```python
from build123d import *

# Parameters (mm, degrees)
F0_R     = 25
F1_DEPTH = 20
F2_R     = 14
F3_DEPTH = 4
F2_R_2   = 25
F2_R_3   = 16.4
F4_DEPTH = 10
F5_SIZE  = 5


with BuildPart() as f1:
    # F0 (on Top) → F1 (new body)
    with BuildSketch(Plane.XY):
        Circle(F0_R)
    extrude(amount=F1_DEPTH)

    # F2 (on face) → F3 (join)
    with BuildSketch(Plane.XY.offset(20)):
        Circle(F2_R)
    extrude(amount=F3_DEPTH)

    # F2 (on face) → F4 (join)
    with BuildSketch(Plane.XY.offset(20)):
        Circle(F2_R_2)
        Circle(F2_R_3, mode=Mode.SUBTRACT)
    extrude(amount=F4_DEPTH)

    # F5
    f5_edges = [f1.edges().sort_by_distance(p)[0] for p in [
        (-25, 0, 0),
    ]]
    chamfer(f5_edges, length=F5_SIZE)


solid = f1.part
```
Input: part model. Units: mm. Frame: model coordinates. A direction names the side the tool comes from. Coordinates: 2 decimals unless noted, no trailing zeros. Write each loop counter-clockwise with the first axis right and the second up, starting at its lowest first coordinate (ties: lowest second). Pieces come first, ordered by that corner, then holes. Notation, with made-up numbers: M 29,28.5 L 52,28.5 A20 cw 52,40.5 Z; hole C 89,77.25 d4. An arc over 180 degrees is marked long. Use one line per item in the form item = value.
Q1. Material intervals for probe 1 along Y at (x, z) = (0, 22.25); probe 2 along Y at (x, z) = (0, 27); probe 3 along X at (y, z) = (-11, 20.25), sorted ascending. Write a range as from..to.
Answer below:
probe_1 = -25..-16.4, -14..14, 16.4..25
probe_2 = -25..-16.4, 16.4..25
probe_3 = -22.45..-12.16, -8.66..8.66, 12.16..22.45
Q2. Draft query along X for faces 3 (the face through (12.932, -5.362, 21.972)), 4 (the face through (0, 0, 24)), 5 (the face through (0, 0, 0)), 6 (the face through (-4.39, -19.76, 0.24)). Return one class per face: released by +X, released by -X, zero draft, split by the parting line, or undercut.
Answer below:
face_3 = undercut
face_4 = undercut
face_5 = zero draft
face_6 = split by the parting line
Q3. First-contact query: pin 1 (6 mm diameter, centred on x = 11, z = 11.5, fed in from +Y); pin 2 (12 mm diameter, centred on y = -12, z = 20, fed in from -X). Flat tips, straight axial feed; report the tip coordinate or a pass-through.
Answer below:
pin_1 = 23.69
pin_2 = -24.27
Q4. Set-up query: faces 1 (the face through (23.846, 7.509, 17.325)), 2 (the face through (12.1, 7.4, 20)). Return all of +Z, -Z, +X, -X, +Y, -Y with unobstructed straight access to the full face (end or side cutting, diameter ignored); none if empty.
Answer below:
face_1 = +Z, -Z
face_2 = +Z
Q5. Section C-C (z = 4). Return loops of the section in (x, y), plus the area to 3 significant figures.
Answer below:
outline = C 0,0 d48
area = 1,810 mm²
Q6. Section A-A (x = 0). Return loops of the section in (y, z).
Answer below:
outline = M -25,5 L -20,0 L 20,0 L 25,5 L 25,30 L 16.4,30 L 16.4,20 L 14,20 L 14,24 L -14,24 L -14,20 L -16.4,20 L -16.4,30 L -25,30 Z
